Autodesk Inventor part; units mm, degrees
ref_plane "YZ Plane" through (0, 0, 0) normal (1, 0, 0) x (0, 1, 0)
ref_plane "XZ Plane" through (0, 0, 0) normal (0, 1, 0) x (-1, 0, 0)
ref_plane "XY Plane" through (0, 0, 0) normal (0, 0, 1) x (1, 0, 0)
sketch "Sketch1" plane through (0, 0, 0) normal (0, 0, 1) x (1, 0, 0)
  line L0 (0, 0) -> (26.416, 0)
  line L1 (26.416, 0) -> (26.416, 19.3294)
  line L2 (26.416, 19.3294) -> (0, 19.3294)
  line L3 (0, 19.3294) -> (0, 0)
  circle A0 centre (5.7658, 2.4638) radius 1.5
  circle A1 centre (19.685, 2.4638) radius 1.5
  line L4 (21.8186, 5.2832) -> (24.2316, 5.2832)
  line L5 (24.2316, 5.2832) -> (24.2316, 17.9832)
  line L6 (24.2316, 17.9832) -> (21.8186, 17.9832)
  line L7 (21.8186, 17.9832) -> (21.8186, 5.2832)
  circle A2 centre (23.0251, 6.5532) radius 0.381
  circle A3 centre (23.0251, 9.0932) radius 0.381
  circle A4 centre (23.0251, 11.6332) radius 0.381
  circle A5 centre (23.0251, 14.1732) radius 0.381
  circle A6 centre (23.0251, 16.7132) radius 0.381
  circle A7 centre (3.175, 14.4018) radius 0.4445
  circle A8 centre (3.175, 11.8618) radius 0.4445
  circle A9 centre (3.175, 9.3218) radius 0.4445
  circle A10 centre (18.593, 9.3218) radius 0.4445
  dimension "d0" = 26.416
  dimension "d1" = 19.3294
  dimension "d2" = 3
  dimension "d3" = 3
  dimension "d4" = 5.7658
  dimension "d5" = 2.4638
  dimension "d6" = 13.9192
  dimension "d7" = 6.731
  dimension "d8" = 2.413
  dimension "d9" = 12.7
  dimension "d10" = 5.2832
  dimension "d11" = 2.1844
  dimension "d12" = 1.27
  dimension "d14" = 2.54
  dimension "d15" = 2.54
  dimension "d16" = 2.54
  dimension "d18" = 1.2065
  dimension "d19" = 2.54
  dimension "d20" = 0.762
  dimension "d21" = 0.762
  dimension "d22" = 0.762
  dimension "d23" = 0.762
  dimension "d24" = 0.762
  dimension "d25" = 0.889
  dimension "d26" = 0.889
  dimension "d27" = 0.889
  dimension "d28" = 4.9276
  dimension "d29" = 2.54
  dimension "d30" = 2.54
  dimension "d31" = 3.175
extrude "Extrusion1" add sketch "Sketch1" along normal blind 1.524 contours L3 L2 L1 L0 | L7 L6 L5 L4 | A10
sketch "Sketch3" plane through (0, 0, 1.524) normal (0, 0, 1) x (1, 0, 0)
  arc A0 (18.9807, 14.6193) -> (18.7439, 13.9837) centre (18.593, 14.4018) ccw
  circle A1 centre (18.593, 9.3218) radius 0.4445
hole "Hole1" at (18.593, 14.4018, 1.524) at (18.593, 9.3218, 1.524) direction (0, 0, -1) diameter 0.889 end through all
equation "\"d26\" = d25"
equation "\"d27\" = d25"
properties part number "pcb"
Can you work these out from the model? Positions are in its coordinate system, mm. Coordinates: 2 decimals unless noted, no trailing zeros. Order: outer loops, then holes, each group sorted by start corner. A loop starts at its lowest first (then second) coordinate and runs counter-clockwise, first axis right, second up. Notation, with made-up numbers: (88, 79.5) - (114, 79.5) arc R7 cw to (114, 87.5) - close; hole circle Ø7 at (40, 50). An arc over 180 degrees is marked (long way). Answer in a Markdown table with one row per item.
1. Suppose I cut it at B-B (z = 1.05). Give the number of separate pieces and of enclosed holes in the cut face, and give its area (3 significant figures).
Reply:
| item | result |
|---|---|
| separate pieces | 1 |
| enclosed holes | 12 |
| area | 491 mm^2 |
2. Suppose I cut it at A-A (x = 6). Please give me the cut outline in (y, z), and give its area (3 significant figures).
Reply:
| item | result |
|---|---|
| outline | (0, 0) - (0.98, 0) - (0.98, 1.52) - (0, 1.52) - close; (3.95, 0) - (19.33, 0) - (19.33, 1.52) - (3.95, 1.52) - close |
| area | 24.9 mm^2 |
3. If I drill on line 1 along Y through (x, z) = (3.5, 1.2); line 2 along X through (y, z) = (1.5, 1.2); line 3 along Y through (x, z) = (22.75, 1.15), over which ranges is the centre line in solid material (lowest first)?
Reply:
| item | result |
|---|---|
| line 1 | y = 0 to 9.02, 9.63 to 11.56, 12.17 to 14.1, 14.71 to 19.33 |
| line 2 | x = 0 to 4.62, 6.92 to 18.54, 20.83 to 26.42 |
| line 3 | y = 0 to 6.29, 6.82 to 8.83, 9.36 to 11.37, 11.9 to 13.91, 14.44 to 16.45, 16.98 to 19.33 |
4. If we mould it in two halves opening along Y, with no side actions, what happens to faces 1 (the cylindrical face through (3.12, 13.96, 0.75)), 2 (the flat face through (13, 10, 1.524)), 3 (the flat face through (13, 0, 1))? For each: pulls with the +Y half, pulls with the -Y half, needs draft (parallel to the pull), parting line crosses it, or undercut.
Reply:
| item | result |
|---|---|
| face 1 | undercut |
| face 2 | needs draft |
| face 3 | pulls with the -Y half |
5. Suppose I cut it at C-C (x = 23). Please give me the cut outline in (y, z).
Reply:
| item | result |
|---|---|
| outline | (0, 0) - (6.17, 0) - (6.17, 1.52) - (0, 1.52) - close; (6.93, 0) - (8.71, 0) - (8.71, 1.52) - (6.93, 1.52) - close; (9.47, 0) - (11.25, 0) - (11.25, 1.52) - (9.47, 1.52) - close; (12.01, 0) - (13.79, 0) - (13.79, 1.52) - (12.01, 1.52) - close; (14.55, 0) - (16.33, 0) - (16.33, 1.52) - (14.55, 1.52) - close; (17.09, 0) - (19.33, 0) - (19.33, 1.52) - (17.09, 1.52) - close |
